The model under review builds one solid part; all positions refer to its coordinate system, in mm. Face numbers are marked on the shaded views. A direction names the side the tool comes from. Round coordinates to 2 decimals unless told otherwise and drop trailing zeros. Write each loop counter-clockwise with the first axis right and the second up, starting at its lowest first coordinate (ties: lowest second). Pieces come first, ordered by that corner, then holes. Notation, with made-up numbers: M 17.5,17.5 L 35.5,17.5 A34 ccw 35.5,53.5 Z; hole C 47,63 d5. An arc over 180 degrees is marked long. Write item = value, one per line. Start each with the question number.
Item 1: To check wall thickness, follow line 1 along X through (y, z) = (7, 8); line 2 along Z through (x, y) = (-8, 7.75) (3 decimals); line 3 along Z through (x, y) = (-12.5, 9). State the ranges of each line that lie inside material, in increasing order.
Item 2: For pin 1 Ø4 at (x, z) = (-13, -3.5) entering from +Y; pin 2 Ø6 at (x, z) = (13, 1.5) entering from -Y; pin 3 Ø1.2 at (x, z) = (-17, -17) entering from +Y; pin 4 Ø2.5 at (x, z) = (17, 17) entering from -Y, all flat-tipped, find the tip position at first contact; note any pin that passes through.
Item 3: The part is to be moulded in two halves that separate along Z. For the marked faces 4, 5 and 6, say which applies: +Z half, -Z half, draft (parallel to the pull), parting line (faces both ways), or undercut.
Item 4: Take a section at A-A, the plane y = 4. Give the boundary of the cut face in (x, z) (3 decimals), plus the area to 3 significant figures.
Item 5: Take a section at D-D, the plane x = -15.5. Give the boundary of the cut face in (y, z), plus the area to 3 significant figures.
Item 6: Tool access review of the marked faces 1, 2 and 3: name each direction out of +Z, -Z, +X, -X, +Y, -Y from which nothing blocks a thin tool from reaching the whole face with its end or side.
Item 7: Take a section at B-B, the plane x = -8. Give the boundary of the cut face in (y, z) (3 decimals), plus the area to 3 significant figures.
Item 8: Take a section at C-C, the plane z = -11.5. Give the boundary of the cut face in (x, y), plus the area to 3 significant figures.
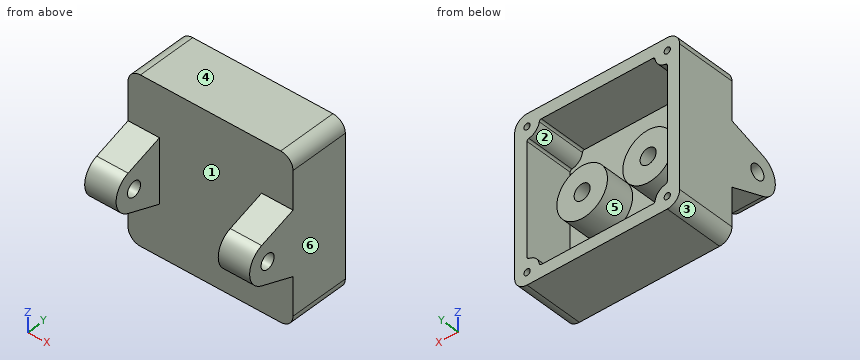
from build123d import *

# Parameters (mm, degrees)
SKETCH1_W           = 40
SKETCH1_H           = 40
BOSS_EXTRUDE1_DEPTH = 2.54
SKETCH2_W           = 40
SKETCH2_H           = 40
BOSS_EXTRUDE2_DEPTH = 12
SKETCH4_R           = 1.813765306
BOSS_EXTRUDE4_DEPTH = 7.62
SKETCH9_R           = 6.145
SKETCH9_R_2         = 1.945
BOSS_EXTRUDE5_DEPTH = 7
FILLET1_R           = 3
SKETCH10_R          = 0.761723834
CUT_EXTRUDE1_DEPTH  = 8


with BuildPart() as part:
    # Sketch1 → Boss-Extrude1 (new body)
    with BuildSketch(Plane(origin=(0, 0, 0), x_dir=(1, 0, 0), z_dir=(0, 1, 0))):
        Rectangle(SKETCH1_W, SKETCH1_H)
    extrude(amount=BOSS_EXTRUDE1_DEPTH)

    # Sketch2 → Boss-Extrude2 (add)
    with BuildSketch(Plane(origin=(0, 2.54, 0), x_dir=(1, 0, 0), z_dir=(0, 1, 0))):
        Rectangle(SKETCH2_W, SKETCH2_H)
        with BuildLine():
            Line((-17, 13.535898385), (-17, -13.535898385))
            ThreePointArc((-17, -13.535898385), (-16.877964473, -13.86322522), (-16.571428571, -14.030770044))
            ThreePointArc((-16.571428571, -14.030770044), (-14.878679656, -14.878679656), (-14.030770044, -16.571428571))
            ThreePointArc((-14.030770044, -16.571428571), (-13.86322522, -16.877964473), (-13.535898385, -17))
            Line((-13.535898385, -17), (13.535898385, -17))
            ThreePointArc((13.535898385, -17), (13.86322522, -16.877964473), (14.030770044, -16.571428571))
            ThreePointArc((14.030770044, -16.571428571), (14.878679656, -14.878679656), (16.571428571, -14.030770044))
            ThreePointArc((16.571428571, -14.030770044), (16.877964473, -13.86322522), (17, -13.535898385))
            Line((17, -13.535898385), (17, 13.535898385))
            ThreePointArc((17, 13.535898385), (16.877964473, 13.86322522), (16.571428571, 14.030770044))
            ThreePointArc((16.571428571, 14.030770044), (14.878679656, 14.878679656), (14.030770044, 16.571428571))
            ThreePointArc((14.030770044, 16.571428571), (13.86322522, 16.877964473), (13.535898385, 17))
            Line((13.535898385, 17), (-13.535898385, 17))
            ThreePointArc((-13.535898385, 17), (-13.86322522, 16.877964473), (-14.030770044, 16.571428571))
            ThreePointArc((-14.030770044, 16.571428571), (-14.878679656, 14.878679656), (-16.571428571, 14.030770044))
            ThreePointArc((-16.571428571, 14.030770044), (-16.877964473, 13.86322522), (-17, 13.535898385))
        make_face(mode=Mode.SUBTRACT)
    extrude(amount=BOSS_EXTRUDE2_DEPTH)

    # Sketch4 → Boss-Extrude4 (add)
    with BuildSketch(Plane.ZY.offset(20)):
        with BuildLine():
            Line((7.748459825, 0), (4.708955343, -8.719310622))
            ThreePointArc((4.708955343, -8.719310622), (0, -12.064660663), (-4.708955343, -8.719310622))
            Line((-4.708955343, -8.719310622), (-7.748459825, 0))
            Line((-7.748459825, 0), (7.748459825, 0))
        make_face()
        with Locations((0, -7.077794281)):
            Circle(SKETCH4_R, mode=Mode.SUBTRACT)
    boss_extrude4 = extrude(amount=-BOSS_EXTRUDE4_DEPTH)

    # Mirror1: Boss-Extrude4 across plane
    add(boss_extrude4.mirror(Plane(origin=(0, 0, 0), x_dir=(0, 0, 1), z_dir=(1, 0, 0))))

    # Sketch9 → Boss-Extrude5 (add)
    with BuildSketch(Plane(origin=(0, 2.54, 0), x_dir=(1, 0, 0), z_dir=(0, 1, 0))):
        with Locations((8, 0)):
            Circle(SKETCH9_R)
        with Locations((8, 0)):
            Circle(SKETCH9_R_2, mode=Mode.SUBTRACT)
        with Locations((-8, 0)):
            Circle(SKETCH9_R)
        with Locations((-8, 0)):
            Circle(SKETCH9_R_2, mode=Mode.SUBTRACT)
    extrude(amount=BOSS_EXTRUDE5_DEPTH)

    # Fillet1
    fillet1_edges = [part.edges().sort_by_distance(p)[0] for p in [
        (20, 7.27, 20),
        (-20, 7.27, 20),
        (-20, 7.27, -20),
        (20, 7.27, -20),
    ]]
    fillet(fillet1_edges, radius=FILLET1_R)

    # Sketch10 → Cut-Extrude1 (cut)
    with BuildSketch(Plane(origin=(0, 14.54, 0), x_dir=(1, 0, 0), z_dir=(0, 1, 0))):
        with Locations((-17, 17)):
            Circle(SKETCH10_R)
        with Locations((17, 17)):
            Circle(SKETCH10_R)
        with Locations((-17, -17)):
            Circle(SKETCH10_R)
        with Locations((17, -17)):
            Circle(SKETCH10_R)
    extrude(amount=-CUT_EXTRUDE1_DEPTH, mode=Mode.SUBTRACT)


solid = part.part
Response values:
q1.line_1 = -20 to -17, 17 to 20
q1.line_2 = -20 to -17, -6.145 to -1.945, 1.945 to 6.145, 17 to 20
q1.line_3 = -20 to -17, -4.18 to 4.18, 17 to 20
q2.pin_1 = 9.54
q2.pin_2 = -12.06
q2.pin_3 = 6.54
q2.pin_4 = 0
q3.face_4 = +Z half
q3.face_5 = undercut
q3.face_6 = draft
q4.outline = M -20,-17 A3 ccw -17,-20 L 17,-20 A3 ccw 20,-17 L 20,17 A3 ccw 17,20 L -17,20 A3 ccw -20,17 Z; C -8,0 d12.29; C 8,0 d12.29; hole M -17,-13.536 A0.5 ccw -16.571,-14.031 A3 cw -14.031,-16.571 A0.5 ccw -13.536,-17 L 13.536,-17 A0.5 ccw 14.031,-16.571 A3 cw 16.571,-14.031 A0.5 ccw 17,-13.536 L 17,13.536 A0.5 ccw 16.571,14.031 A3 cw 14.031,16.571 A0.5 ccw 13.536,17 L -13.536,17 A0.5 ccw -14.031,16.571 A3 cw -16.571,14.031 A0.5 ccw -17,13.536 Z; hole C -8,0 d3.89; hole C 8,0 d3.89
q4.area = 678 mm2
q5.outline = M -8.72,-4.71 L 0,-7.75 L 0,-20 L 14.54,-20 L 14.54,-14.4 L 2.54,-14.4 L 2.54,14.4 L 14.54,14.4 L 14.54,20 L 0,20 L 0,7.75 L -8.72,4.71 A4.99 ccw Z; hole C -7.08,0 d3.63
q5.area = 357 mm2
q6.face_1 = -Y
q6.face_2 = +Y
q6.face_3 = -Z, -X, +Y, -Y
q7.outline = M 0,-20 L 14.54,-20 L 14.54,-17 L 2.54,-17 L 2.54,-6.145 L 9.54,-6.145 L 9.54,-1.945 L 2.54,-1.945 L 2.54,1.945 L 9.54,1.945 L 9.54,6.145 L 2.54,6.145 L 2.54,17 L 14.54,17 L 14.54,20 L 0,20 Z
q7.area = 232 mm2
q8.outline = M -20,0 L 20,0 L 20,14.54 L 17,14.54 L 17,2.54 L -17,2.54 L -17,14.54 L -20,14.54 Z
q8.area = 174 mm2
